Part model, mm, in its own coordinate system. A direction names the side the tool comes from. Give positions to 0.01 mm unless a question says otherwise; leave off trailing zeros. Order: outer loops, then holes, each group sorted by start corner. A loop starts at its lowest first (then second) coordinate and runs counter-clockwise, first axis right, second up. Notation, with made-up numbers: (3, -35) -> (22, -35) arc R24 ccw to (22, -9) -> close; hole circle Ø3 at (78, 25). An arc over 180 degrees is marked (long way). Write item = value, one per line. Start each with the question number.
Item 1: Band-saw the part on D-D on x = 28. Write the cut outline in (y, z), plus the area to 3 significant figures.
Item 2: Band-saw the part on B-B on y = 93.74. Write the cut outline in (x, z).
Item 3: Band-saw the part on A-A on x = 20. Write the cut outline in (y, z), plus the area to 3 significant figures.
Item 4: Tool access for faces 4 (the face through (10, 50, 17)), 5 (the face through (40, 32, 13)), 6 (the face through (21.494, 32.417, 16.836)), 7 (the face through (20, 125.31, 32)), 8 (the face through (3.5, 33, 17)): list every direction of +Z, -Z, +X, -X, +Y, -Y with a clear straight run to the whole face (end or side of a thin tool).
Item 5: Band-saw the part on C-C on z = 3. Write the cut outline in (x, y), plus the area to 3 significant figures.
Item 6: Pull direction Y, two halves, no side cores. Call faces 1 (the face through (20, 8, 21.5)), 2 (the face through (50.07, 61.6, 17.74)), 3 (the face through (42.985, 67.534, 32.042)): +Y half, -Y half, draft (parallel to the pull), parting line (faces both ways), or undercut.
Item 7: Drill centre lines: line 1 along Y through (x, z) = (43.57, 31); line 2 along Y through (x, z) = (11, 26); line 3 along Y through (x, z) = (20, 7.5). Where is each one in solid material? Low to high.
Item 8: Flat gauge pins, fed straight in: P1, Ø2.5, axis at x = 50, z = 21.5, coming from the +Y side; P2, Ø1, axis at y = 61.5, z = 6, coming from the -X side; P3, Ø9, axis at y = 27.36, z = 17.5, coming from the +X side; P4, Ø5.5, axis at x = 43, z = 25, coming from the -Y side. Where does each tip first touch, or does it go through?
```python
from build123d import *

# Parameters (mm, degrees)
CROQUIS1_R                   = 3.25
SALIENTE_EXTRUIR1_DEPTH      = 35
CROQUIS3_R                   = 5.1
CROQUIS3_W                   = 8
CROQUIS3_H                   = 16.86
CORTAR_EXTRUIR2_DEPTH        = 85.095950556
CROQUIS4_R                   = 11
CORTAR_EXTRUIR3_DEPTH        = 3.5
CROQUIS5_R                   = 20
CROQUIS5_R_2                 = 2.7
SALIENTE_EXTRUIR3_DEPTH      = 6
SALIENTE_EXTRUIR5_DEPTH      = 29
SALIENTE_EXTRUIR5_DEPTH_BACK = 6
CROQUIS9_W                   = 56.4
CROQUIS9_H                   = 56.4
CORTAR_EXTRUIR4_DEPTH        = 29


with BuildPart() as part:
    # Croquis1 → Saliente-Extruir1 (new body)
    # profile 1 of 2: a face of its own
    with BuildSketch(Plane.XY):
        with BuildLine():
            Line((0, 60.17), (0, 40.17))
            Line((0, 40.17), (10, 40.17))
            Line((10, 40.17), (10, 60.17))
            Line((10, 60.17), (30, 60.17))
            Line((30, 60.17), (30, 40.17))
            Line((30, 40.17), (40, 40.17))
            Line((40, 40.17), (40, 60.17))
            ThreePointArc((40, 60.17), (38.535533906, 63.705533906), (35, 65.17))
            Line((35, 65.17), (5, 65.17))
            ThreePointArc((5, 65.17), (1.464466094, 63.705533906), (0, 60.17))
        make_face()
    # profile 2 of 2: a face of its own
    with BuildSketch(Plane.XY):
        with BuildLine():
            Line((5, 0), (35, 0))
            ThreePointArc((35, 0), (38.535533906, 1.464466094), (40, 5))
            Line((40, 5), (40, 40.17))
            Line((40, 40.17), (0, 40.17))
            Line((0, 40.17), (0, 5))
            ThreePointArc((0, 5), (1.464466094, 1.464466094), (5, 0))
        make_face()
        with Locations((20, 4)):
            Circle(CROQUIS1_R, mode=Mode.SUBTRACT)
    extrude(amount=SALIENTE_EXTRUIR1_DEPTH)

    # Croquis3 → Cortar-Extruir2 (cut, through all)
    with BuildSketch(Plane.ZY):
        with Locations((17.5, 27.36)):
            Circle(CROQUIS3_R)
        with Locations((17.5, 8.43)):
            Rectangle(CROQUIS3_W, CROQUIS3_H)
    extrude(amount=-CORTAR_EXTRUIR2_DEPTH, mode=Mode.SUBTRACT)

    # Croquis4 → Cortar-Extruir3 (cut)
    with BuildSketch(Plane.ZY):
        with Locations((17.5, 27.36)):
            Circle(CROQUIS4_R)
    extrude(amount=-CORTAR_EXTRUIR3_DEPTH, mode=Mode.SUBTRACT)

    # Croquis5 → Saliente-Extruir3 (add)
    with BuildSketch(Plane.XY.offset(35)):
        with BuildLine():
            Line((-11.57, 120.31), (-11.57, 67.17))
            ThreePointArc((-11.57, 67.17), (-10.105533906, 63.634466094), (-6.57, 62.17))
            Line((-6.57, 62.17), (46.57, 62.17))
            ThreePointArc((46.57, 62.17), (50.105533906, 63.634466094), (51.57, 67.17))
            Line((51.57, 67.17), (51.57, 120.31))
            ThreePointArc((51.57, 120.31), (50.105533906, 123.845533906), (46.57, 125.31))
            Line((46.57, 125.31), (-6.57, 125.31))
            ThreePointArc((-6.57, 125.31), (-10.105533906, 123.845533906), (-11.57, 120.31))
        make_face()
        with Locations((20, 93.74)):
            Circle(CROQUIS5_R, mode=Mode.SUBTRACT)
        with Locations((-3.57, 117.31)):
            Circle(CROQUIS5_R_2, mode=Mode.SUBTRACT)
        with Locations((43.57, 117.31)):
            Circle(CROQUIS5_R_2, mode=Mode.SUBTRACT)
        with Locations((43.57, 70.17)):
            Circle(CROQUIS5_R_2, mode=Mode.SUBTRACT)
        with Locations((-3.57, 70.17)):
            Circle(CROQUIS5_R_2, mode=Mode.SUBTRACT)
    extrude(amount=-SALIENTE_EXTRUIR3_DEPTH)

    # Croquis8 → Saliente-Extruir5 (add, two sides: drawn at the far end of the back side and taken through both)
    with BuildSketch(Plane(origin=(0, 0, 29), x_dir=(-1, 0, 0), z_dir=(0, 0, -1)).offset(-SALIENTE_EXTRUIR5_DEPTH_BACK)):
        with BuildLine():
            Line((6.57, 60.17), (-46.57, 60.17))
            ThreePointArc((-46.57, 60.17), (-50.105533906, 61.634466094), (-51.57, 65.17))
            Line((-51.57, 65.17), (-51.57, 67.17))
            Line((-51.57, 67.17), (11.57, 67.17))
            Line((11.57, 67.17), (11.57, 65.17))
            ThreePointArc((11.57, 65.17), (10.105533906, 61.634466094), (6.57, 60.17))
        make_face()
    extrude(amount=SALIENTE_EXTRUIR5_DEPTH + SALIENTE_EXTRUIR5_DEPTH_BACK)

    # Croquis9 → Cortar-Extruir4 (cut)
    with BuildSketch(Plane(origin=(0, 0, 0), x_dir=(-1, 0, 0), z_dir=(0, 0, -1))):
        with Locations((-20, 93.74)):
            Rectangle(CROQUIS9_W, CROQUIS9_H)
    extrude(amount=-CORTAR_EXTRUIR4_DEPTH, mode=Mode.SUBTRACT)


solid = part.part
```
Values found:
q1.outline = (0, 0) -> (40.17, 0) -> (40.17, 35) -> (0, 35) -> (0, 21.5) -> (16.86, 21.5) -> (16.86, 13.5) -> (0, 13.5) -> close; (60.17, 0) -> (65.54, 0) -> (65.54, 29) -> (75.41, 29) -> (75.41, 35) -> (60.17, 35) -> close; (112.07, 29) -> (125.31, 29) -> (125.31, 35) -> (112.07, 35) -> close; hole circle Ø10.2 at (27.36, 17.5)
q1.area = 1,520 mm^2
q2.outline = (-11.57, 29) -> (0, 29) -> (0, 35) -> (-11.57, 35) -> close; (40, 29) -> (51.57, 29) -> (51.57, 35) -> (40, 35) -> close
q3.outline = (0, 0) -> (0.75, 0) -> (0.75, 13.5) -> (0, 13.5) -> close; (0, 21.5) -> (0.75, 21.5) -> (0.75, 35) -> (0, 35) -> close; (7.25, 0) -> (40.17, 0) -> (40.17, 35) -> (7.25, 35) -> (7.25, 21.5) -> (16.86, 21.5) -> (16.86, 13.5) -> (7.25, 13.5) -> close; (60.17, 0) -> (65.54, 0) -> (65.54, 29) -> (73.74, 29) -> (73.74, 35) -> (60.17, 35) -> close; (113.74, 29) -> (125.31, 29) -> (125.31, 35) -> (113.74, 35) -> close; hole circle Ø10.2 at (27.36, 17.5)
q3.area = 1,320 mm^2
q4.face_4 = +Z, -Z
q4.face_5 = +Z, -Z, +X, -Y
q4.face_6 = +X, -X
q4.face_7 = +Z, -Z, +X, -X, +Y
q4.face_8 = -X
q5.outline = (-11.57, 65.17) arc R5 ccw to (-6.57, 60.17) -> (0, 60.17) -> (0, 5) arc R5 ccw to (5, 0) -> (35, 0) arc R5 ccw to (40, 5) -> (40, 60.17) -> (46.57, 60.17) arc R5 ccw to (51.57, 65.17) -> (51.57, 67.17) -> (48.2, 67.17) -> (48.2, 65.54) -> (-8.2, 65.54) -> (-8.2, 67.17) -> (-11.57, 67.17) -> close; hole (10, 40.17) -> (30, 40.17) -> (30, 60.17) -> (10, 60.17) -> close; hole circle Ø6.5 at (20, 4)
q5.area = 2,300 mm^2
q6.face_1 = draft
q6.face_2 = -Y half
q6.face_3 = undercut
q7.line_1 = 60.17 to 67.47, 72.87 to 114.61, 120.01 to 125.31
q7.line_2 = 0 to 40.17, 60.17 to 65.54
q7.line_3 = 0 to 0.75, 7.25 to 40.17, 60.17 to 65.54
q8.P1 = 67.17
q8.P2 = -10.44
q8.P3 = through
q8.P4 = 60.17
